```python
from build123d import *

# Parameters (mm, degrees)
F0_R     = 25.357029
F1_DEPTH = 80
F2_R     = 19
F3_DEPTH = 99.8
F5_R     = 21.659123
F6_DEPTH = 2


with BuildPart() as f1:
    # F0 (on Front) → F1 (new body)
    with BuildSketch(Plane.XZ):
        Circle(F0_R)
    extrude(amount=-F1_DEPTH)

    # F2 (on face) → F3 (cut)
    with BuildSketch(Plane.XZ):
        Circle(F2_R)
    extrude(amount=-F3_DEPTH, mode=Mode.SUBTRACT)

    # F5 (on offset) → F6 (cut)
    with BuildSketch(Plane.XZ.offset(-34.4)):
        Circle(F5_R)
    extrude(amount=-F6_DEPTH, mode=Mode.SUBTRACT)


solid = f1.part
```
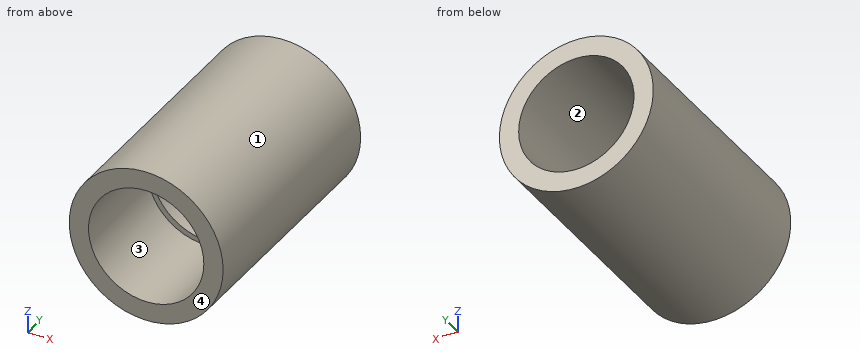
The model under review builds one solid part; all positions refer to its coordinate system, in mm. Face numbers are marked on the shaded views. Round coordinates to 2 decimals unless told otherwise and drop trailing zeros. Loops run counter-clockwise (first coordinate to the right, second up) from the corner with the lowest first, then second, coordinate; pieces in that order, holes last.
1) Consider section D-D on y = 69. State the section outline as (x, z) points, then the cut area to 3 significant figures.
Values follow:
outline: circle Ø50.71 at (0, 0); hole circle Ø38 at (0, 0)
area: 886 mm2
2) The part is to be moulded in two halves that separate along Z. For the marked faces 1, 2, 3 and 4, say which applies: pulls with the +Z half, pulls with the -Z half, needs draft (parallel to the pull), parting line crosses it, or undercut.
Values follow:
face 1: parting line crosses it
face 2: undercut
face 3: undercut
face 4: needs draft
3) Clearance check with flat-ended pins moving along their axes: P1, Ø4, axis at y = 23.5, z = 9.5, coming from the +X side; P2, Ø23, axis at x = 0, z = 0, coming from the +Y side; P3, Ø10, axis at x = -10.5, y = 59, coming from the -Z side; P4, Ø8, axis at x = -13, y = 16.5, coming from the +Z side. State where each tip first meets the part, or that it passes through.
Values follow:
P1: stops at x = 24.22
P2: passes through
P3: stops at z = -24.75
P4: stops at z = 23.71
4) Consider section C-C on x = 20. State the section outline as (y, z) points.
Values follow:
outline: (0, -15.59) - (80, -15.59) - (80, 15.59) - (0, 15.59) - close; hole (34.4, -8.31) - (36.4, -8.31) - (36.4, 8.31) - (34.4, 8.31) - close
5) Consider section A-A on x = 0. State the section outline as (y, z) points, then the cut area to 3 significant figures.
Values follow:
outline: (0, -25.36) - (80, -25.36) - (80, -19) - (36.4, -19) - (36.4, -21.66) - (34.4, -21.66) - (34.4, -19) - (0, -19) - close; (0, 19) - (34.4, 19) - (34.4, 21.66) - (36.4, 21.66) - (36.4, 19) - (80, 19) - (80, 25.36) - (0, 25.36) - close
area: 1,010 mm2
6) Wall thickness on line 1 along Y through (x, z) = (17, 11); line 2 along Z through (x, y) = (0, 67); line 3 along X through (y, z) = (13, -7): over which ranges is each line inside the solid? List them lowest first.
Values follow:
line 1: y = 0 to 34.4, 36.4 to 80
line 2: z = -25.36 to -19, 19 to 25.36
line 3: x = -24.37 to -17.66, 17.66 to 24.37
7) Consider section B-B on z = 0. State the section outline as (x, y) points.
Values follow:
outline: (-25.36, 0) - (-19, 0) - (-19, 34.4) - (-21.66, 34.4) - (-21.66, 36.4) - (-19, 36.4) - (-19, 80) - (-25.36, 80) - close; (19, 0) - (25.36, 0) - (25.36, 80) - (19, 80) - (19, 36.4) - (21.66, 36.4) - (21.66, 34.4) - (19, 34.4) - close
